Geometry check sheet. Reference: the model listing, model coordinates, mm. A direction names the side the tool comes from. Coordinates: 2 decimals unless noted, no trailing zeros. Order: outer loops, then holes, each group sorted by start corner. A loop starts at its lowest first (then second) coordinate and runs counter-clockwise, first axis right, second up.
```python
from build123d import *

# Parameters (mm, degrees)
BOSS_EXTRUDE1_DEPTH     = 52.5
SKETCH2_R               = 7
CUT_EXTRUDE1_DEPTH      = 105
BOSS_EXTRUDE2_REACH     = 58.735
SKETCH5_R               = 14.397777867
BOSS_EXTRUDE3_REACH     = 58.735
SKETCH5_2_R             = 14.397777867
SKETCH7_R               = 10.5
CUT_EXTRUDE2_DEPTH      = 75
CUT_EXTRUDE2_DEPTH_BACK = 116
FILLET1_R               = 5


with BuildPart() as part:
    # Sketch1 → Boss-Extrude1 (new body, symmetric)
    with BuildSketch(Plane(origin=(0, 0, 0), x_dir=(0, 0, -1), z_dir=(1, 0, 0))):
        Polygon((-32.5, 0), (32.5, 0), (32.5, -16), (15.5, -16), (15.5, -32), (-15.5, -32), (-15.5, -16), (-32.5, -16), align=None)
    extrude(amount=BOSS_EXTRUDE1_DEPTH, both=True)

    # Sketch2 → Cut-Extrude1 (cut)
    with BuildSketch(Plane(origin=(0, 0, 0), x_dir=(1, 0, 0), z_dir=(0, 1, 0))):
        with Locations((37.5, 0)):
            Circle(SKETCH2_R)
        with Locations((-37.5, 0)):
            Circle(SKETCH2_R)
    extrude(amount=-CUT_EXTRUDE1_DEPTH, mode=Mode.SUBTRACT)

    # Boss-Extrude2: up to this face of the body (flat: up to its plane)
    boss_extrude2_end = Plane(part.part.faces().sort_by_distance((0, -8, 32.5))[0])
    # Sketch5 → Boss-Extrude2 (add, up to the picked face)
    with BuildSketch(Plane(origin=(0, 0, 0), x_dir=(0.819152044, 0, 0.573576436), z_dir=(-0.573576436, 0, 0.819152044)), mode=Mode.PRIVATE) as boss_extrude2_sk1:
        Circle(SKETCH5_R)
    boss_extrude2_tool1 = split(extrude(boss_extrude2_sk1.sketch, amount=BOSS_EXTRUDE2_REACH, mode=Mode.PRIVATE), bisect_by=boss_extrude2_end, keep=Keep.BOTH, mode=Mode.PRIVATE)
    add(boss_extrude2_tool1.solids().sort_by_distance((0, 0, 0))[0])

    # Boss-Extrude3: up to this face of the body (flat: up to its plane)
    boss_extrude3_end = Plane(part.part.faces().sort_by_distance((0, -8, -32.5))[0])
    # Sketch5<2> → Boss-Extrude3 (add, up to the picked face)
    with BuildSketch(Plane(origin=(0, 0, 0), x_dir=(0.819152044, 0, 0.573576436), z_dir=(-0.573576436, 0, 0.819152044)), mode=Mode.PRIVATE) as boss_extrude3_sk1:
        Circle(SKETCH5_2_R)
    boss_extrude3_tool1 = split(extrude(boss_extrude3_sk1.sketch, amount=-BOSS_EXTRUDE3_REACH, mode=Mode.PRIVATE), bisect_by=boss_extrude3_end, keep=Keep.BOTH, mode=Mode.PRIVATE)
    add(boss_extrude3_tool1.solids().sort_by_distance((0, 0, 0))[0])

    # Sketch7 → Cut-Extrude2 (cut, two sides)
    with BuildSketch(Plane(origin=(0, 0, 0), x_dir=(0.819152044, 0, 0.573576436), z_dir=(-0.573576436, 0, 0.819152044))) as cut_extrude2_sk:
        Circle(SKETCH7_R)
    extrude(amount=CUT_EXTRUDE2_DEPTH, mode=Mode.SUBTRACT)
    extrude(cut_extrude2_sk.sketch, amount=-CUT_EXTRUDE2_DEPTH_BACK, mode=Mode.SUBTRACT)

    # Fillet1
    fillet1_edges = [part.edges().sort_by_distance(p)[0] for p in [
        (17.576441355, 0, 0),
        (-17.576441355, 0, 0),
    ]]
    fillet(fillet1_edges, radius=FILLET1_R)


solid = part.part
```
Item 1: Thickness scan on line 1 along X through (y, z) = (-12, 0); line 2 along Z through (x, y) = (37.5, -12); line 3 along Z through (x, y) = (-37.5, -21). Record the ranges inside material, lowest first.
Item 2: Sectioned sample at A-A (y = -8.5). Record the cut outline in (x, z), and give its area (3 significant figures).
Item 3: Sectioned sample at C-C (y = -20). Record the cut outline in (x, z), and give its area (3 significant figures).
Item 4: Tool access check on faces 1 (the face through (1, -16, 24)), 2 (the face through (-32, 0, -7)), 3 (the face through (1, -24, -15.5)), 4 (the face through (32, 0, 8)). Record the directions out of +Z, -Z, +X, -X, +Y, -Y that give a thin tool (end or side, any length) a straight path to the whole face; none if there is none.
Item 5: Sectioned sample at B-B (z = 4.5). Give the number of separate pieces and of enclosed holes in the cut face, and give its area (3 significant figures).
Item 6: Release check for a two-part mould opening along Z. For faces 5 (the face through (7.74, 3.15, 6.41)), 6 (the face through (1, -24, 15.5)), 7 (the face through (1, -16, -24)) record: pulls with the +Z half, pulls with the -Z half, needs draft (parallel to the pull), parting line crosses it, or undercut.
Item 7: Depth check by flat-ended pin: P1, Ø1, axis at x = -40.5, z = 18, coming from the +Y side; P2, Ø18.5, axis at x = -11.5, z = -25.5, coming from the -Y side; P3, Ø1.5, axis at x = 31, y = -18.5, coming from the -Z side; P4, Ø8.5, axis at x = 37.5, z = 0, coming from the +Y side. Enter the tip coordinate at first touch or a pass-through.
Geometry check:
1. line 1: x = -52.5 to -44.5, -30.5 to 30.5, 44.5 to 52.5
1. line 2: z = -32.5 to -7, 7 to 32.5
1. line 3: z = -15.5 to -7, 7 to 15.5
2. outline: (-52.5, -32.5) - (15.23, -32.5) - (-30.28, 32.5) - (-52.5, 32.5) - close; (-15.23, 32.5) - (30.28, -32.5) - (52.5, -32.5) - (52.5, 32.5) - close; hole circle Ø14 at (-37.5, 0); hole circle Ø14 at (37.5, 0)
2. area: 5,540 mm2
3. outline: (-52.5, -15.5) - (52.5, -15.5) - (52.5, 15.5) - (-52.5, 15.5) - close; hole circle Ø14 at (-37.5, 0); hole circle Ø14 at (37.5, 0)
3. area: 2,950 mm2
4. face 1: +Z, +X, -X, -Y
4. face 2: -Z, -X, +Y
4. face 3: -Z, +X, -X, -Y
4. face 4: +Z, +X, +Y
5. separate pieces: 3
5. enclosed holes: 1
5. area: 2,660 mm2
6. face 5: undercut
6. face 6: pulls with the +Z half
6. face 7: needs draft
7. P1: stops at y = 0
7. P2: stops at y = -16
7. P3: stops at z = -15.5
7. P4: passes through
